Check sheet for the modelled part. Datum: model origin and axes. Units: mm. Face numbers are marked on the shaded views. A direction names the side the tool comes from. Coordinates: 2 decimals unless noted, no trailing zeros. Write each loop counter-clockwise with the first axis right and the second up, starting at its lowest first coordinate (ties: lowest second). Pieces come first, ordered by that corner, then holes. Notation, with made-up numbers: (-40, 35) -> (-16, 35) arc R21 ccw to (-16, 71) -> close; hole circle Ø5 at (52, -39.5). An arc over 180 degrees is marked (long way). Put each result on its own line as item: value.
```python
from build123d import *

# Parameters (mm, degrees)
SKETCH1_W           = 115
SKETCH1_H           = 110
BOSS_EXTRUDE1_DEPTH = 45
SKETCH2_W           = 110
SKETCH2_H           = 105
CUT_EXTRUDE1_DEPTH  = 40
SKETCH10_R          = 5
BOSS_EXTRUDE4_DEPTH = 11
SKETCH11_R          = 1
CUT_EXTRUDE8_DEPTH  = 85.689137438
CUT_EXTRUDE9_REACH  = 134.027
SKETCH14_W          = 35
SKETCH14_H          = 18
SKETCH16_W          = 12
SKETCH16_H          = 60
CUT_EXTRUDE10_DEPTH = 5


with BuildPart() as part:
    # Sketch1 → Boss-Extrude1 (new body)
    with BuildSketch(Plane.XY):
        Rectangle(SKETCH1_W, SKETCH1_H)
    extrude(amount=BOSS_EXTRUDE1_DEPTH)

    # Sketch2 → Cut-Extrude1 (cut)
    with BuildSketch(Plane.XY.offset(45)):
        Rectangle(SKETCH2_W, SKETCH2_H)
    extrude(amount=-CUT_EXTRUDE1_DEPTH, mode=Mode.SUBTRACT)

    # Sketch10 → Boss-Extrude4 (add)
    with BuildSketch(Plane.XY.offset(5)):
        with Locations(Location((-47, -44.5, 0), (0, 0, 180))):
            Circle(SKETCH10_R)
        with Locations(Location((18, -44.5, 0), (0, 0, 180))):
            Circle(SKETCH10_R)
        with Locations(Location((-47, 44.5, 0), (0, 0, 180))):
            Circle(SKETCH10_R)
        with Locations(Location((18, 44.5, 0), (0, 0, 180))):
            Circle(SKETCH10_R)
    extrude(amount=BOSS_EXTRUDE4_DEPTH)

    # Sketch11 → Cut-Extrude8 (cut, through all)
    with BuildSketch(Plane.XY.offset(16)):
        with Locations((-47, 44.5)):
            Circle(SKETCH11_R)
        with Locations((18, 44.5)):
            Circle(SKETCH11_R)
        with Locations((18, -44.5)):
            Circle(SKETCH11_R)
        with Locations((-47, -44.5)):
            Circle(SKETCH11_R)
    extrude(amount=-CUT_EXTRUDE8_DEPTH, mode=Mode.SUBTRACT)

    # Sketch14 → Cut-Extrude9 (cut, up to next)
    with BuildSketch(Plane.XZ.offset(55), mode=Mode.PRIVATE) as cut_extrude9_sk1:
        with Locations((-4.5, 31)):
            Rectangle(SKETCH14_W, SKETCH14_H)
    cut_extrude9_tool1 = extrude(cut_extrude9_sk1.sketch, amount=-CUT_EXTRUDE9_REACH, mode=Mode.PRIVATE) & part.part
    add(cut_extrude9_tool1.solids().sort_by_distance((-4.5, -55, 31))[0], mode=Mode.SUBTRACT)

    # Sketch16 → Cut-Extrude10 (cut)
    with BuildSketch(Plane.ZY.offset(57.5)):
        with Locations((12, 2.5)):
            Rectangle(SKETCH16_W, SKETCH16_H)
    extrude(amount=-CUT_EXTRUDE10_DEPTH, mode=Mode.SUBTRACT)


solid = part.part
```
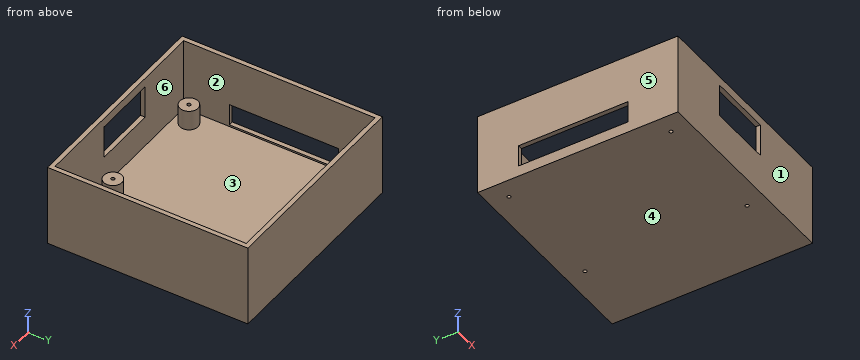
Q1. Material ranges on line 1 along Y through (x, z) = (18, 12); line 2 along X through (y, z) = (-34, 35.5); line 3 along X through (y, z) = (-44, 3), recorded low to high.
Recorded:
line 1: y = -55 to -52.5, -49.5 to -45.5, -43.5 to -39.5, 39.5 to 43.5, 45.5 to 49.5, 52.5 to 55
line 2: x = -57.5 to -55, 55 to 57.5
line 3: x = -57.5 to -47.87, -46.13 to 17.13, 18.87 to 57.5
Q2. Cross-section at A-A (x = -11). Record the cut outline in (y, z), plus the area to 3 significant figures.
Recorded:
outline: (-55, 0) -> (55, 0) -> (55, 45) -> (52.5, 45) -> (52.5, 5) -> (-52.5, 5) -> (-52.5, 22) -> (-55, 22) -> close; (-55, 40) -> (-52.5, 40) -> (-52.5, 45) -> (-55, 45) -> close
area: 705 mm2
Q3. Cross-section at B-B (z = 11.5). State how many separate pieces and enclosed holes the cut face has, plus the area to 3 significant figures.
Recorded:
separate pieces: 5
enclosed holes: 4
area: 1,250 mm2
Q4. Cross-section at C-C (y = 19.5). Record the cut outline in (x, z), plus the area to 3 significant figures.
Recorded:
outline: (-57.5, 0) -> (57.5, 0) -> (57.5, 45) -> (55, 45) -> (55, 5) -> (-55, 5) -> (-55, 6) -> (-57.5, 6) -> close; (-57.5, 18) -> (-55, 18) -> (-55, 45) -> (-57.5, 45) -> close
area: 745 mm2
Q5. Depth check by flat-ended pin: P1, Ø3, axis at x = -45, y = 46.5, coming from the +Z side; P2, Ø1, axis at x = 17, y = 26, coming from the +Z side. Enter the tip coordinate at first touch or a pass-through.
Recorded:
P1: stops at z = 16
P2: stops at z = 5
Q6. Mould release check, pull along X, two halves, no side actions. Record for the marked faces 3, 4, 5 and 6: released by +X, released by -X, zero draft, split by the parting line, or undercut.
Recorded:
face 3: undercut
face 4: zero draft
face 5: released by -X
face 6: undercut
Q7. Cross-section at D-D (x = 38.5). Record the cut outline in (y, z).
Recorded:
outline: (-55, 0) -> (55, 0) -> (55, 45) -> (52.5, 45) -> (52.5, 5) -> (-52.5, 5) -> (-52.5, 45) -> (-55, 45) -> close
Q8. Tool access check on the marked faces 1 and 2. Record the directions out of +Z, -Z, +X, -X, +Y, -Y that give a thin tool (end or side, any length) a straight path to the whole face; none if there is none.
Recorded:
face 1: +Z, -Z, +X, -X, -Y
face 2: +Z
